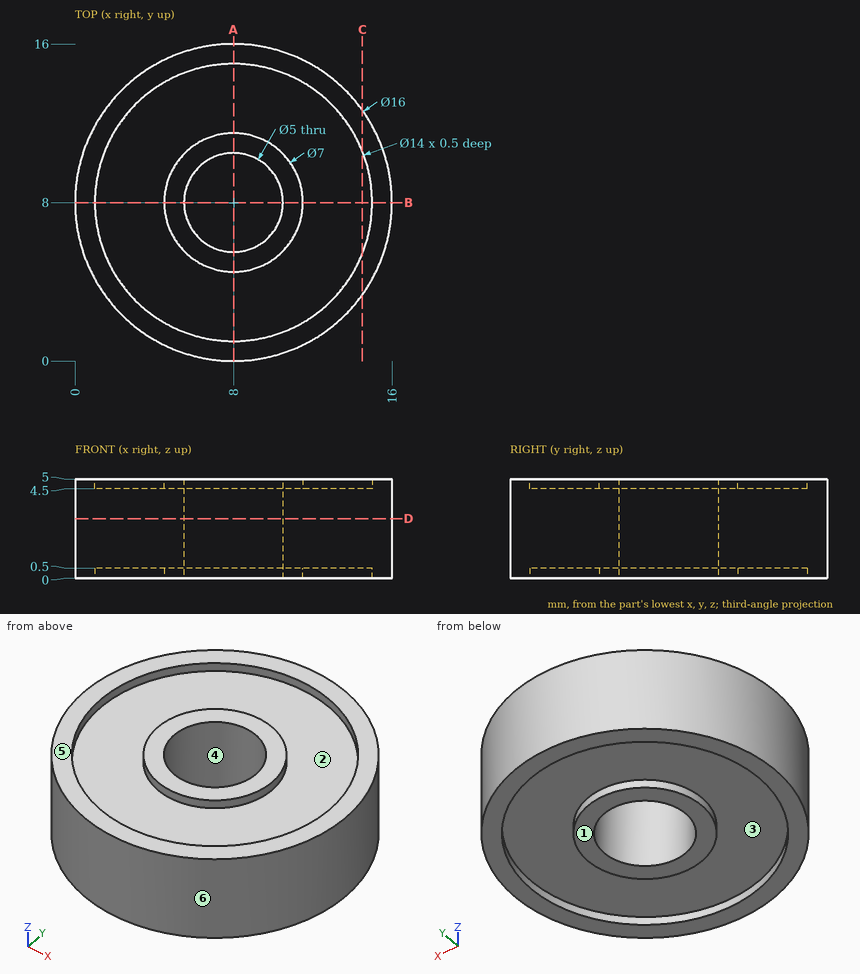
Design review of the part shown in the three views and the two pictorial views. Dimensions are in mm from the part's minimum x, y and z. A direction names the side the tool comes from. Round coordinates to 2 decimals unless told otherwise and drop trailing zeros. Loops run counter-clockwise (first coordinate to the right, second up) from the corner with the lowest first, then second, coordinate; pieces in that order, holes last.
Q1. To check wall thickness, follow line 1 along Y through (x, z) = (7.25, 4.85); line 2 along Y through (x, z) = (8, 0.45); line 3 along Y through (x, z) = (8, 2.7). State the ranges of each line that lie inside material, in increasing order.
Result sheet:
line 1: y = 0.04 to 1.04, 4.58 to 5.62, 10.38 to 11.42, 14.96 to 15.96
line 2: y = 0 to 1, 4.5 to 5.5, 10.5 to 11.5, 15 to 16
line 3: y = 0 to 5.5, 10.5 to 16
Q2. Add section D-D on z = 3. Write out the cut boundary in (x, y).
Result sheet:
outline: circle Ø16 at (8, 8); hole circle Ø5 at (8, 8)
Q3. Machinability: for the marked faces 1 and 2, which of the approach directions +Z, -Z, +X, -X, +Y, -Y give a long, thin tool a straight path to every point of the face, cutting with its end or side? Answer none if there is none.
Result sheet:
face 1: -Z, +X, -X, +Y, -Y
face 2: +Z
Q4. Add section A-A on x = 8. Write out the cut boundary in (y, z), plus the area to 3 significant figures.
Result sheet:
outline: (0, 0) - (1, 0) - (1, 0.5) - (4.5, 0.5) - (4.5, 0) - (5.5, 0) - (5.5, 5) - (4.5, 5) - (4.5, 4.5) - (1, 4.5) - (1, 5) - (0, 5) - close; (10.5, 0) - (11.5, 0) - (11.5, 0.5) - (15, 0.5) - (15, 0) - (16, 0) - (16, 5) - (15, 5) - (15, 4.5) - (11.5, 4.5) - (11.5, 5) - (10.5, 5) - close
area: 48.0 mm2
Q5. Add section C-C on x = 14.5. Write out the cut boundary in (y, z), plus the area to 3 significant figures.
Result sheet:
outline: (3.34, 0) - (5.4, 0) - (5.4, 0.5) - (10.6, 0.5) - (10.6, 0) - (12.66, 0) - (12.66, 5) - (10.6, 5) - (10.6, 4.5) - (5.4, 4.5) - (5.4, 5) - (3.34, 5) - close
area: 41.4 mm2
Q6. Mouldability with a two-part tool opening along Y and no side actions: class the marked faces 3, 4, 5 and 6 as +Y half, -Y half, draft (parallel to the pull), parting line (faces both ways), or undercut.
Result sheet:
face 3: undercut
face 4: undercut
face 5: draft
face 6: parting line
Q7. Insertion check: pin 1 Ø4 at (x, y) = (5.5, 10.5) entering from +Z. The pin has a flat end and moves straight along its axis. Give the tip position at first contact, or say it passes through.
Result sheet:
pin 1: stops at z = 5
